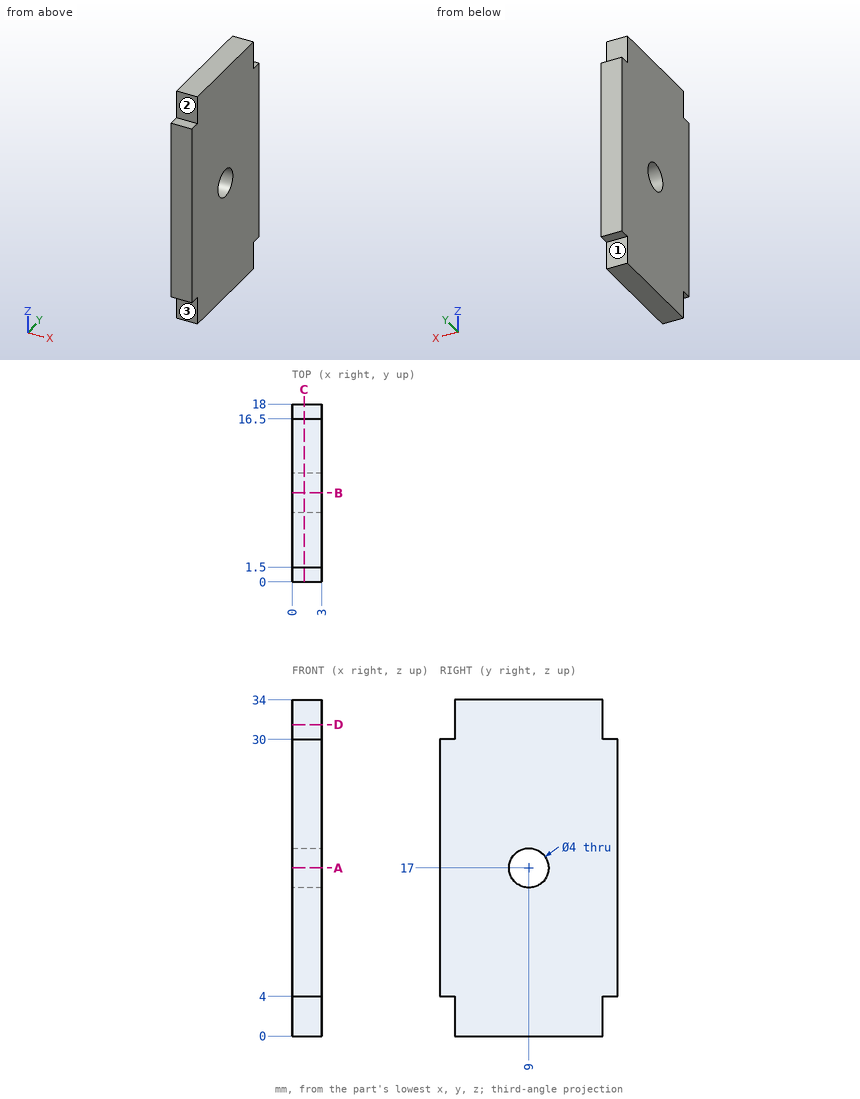
Drawing for the job (mm, zero at the part's lowest x, y, z). A direction names the side the tool comes from. Round coordinates to 2 decimals unless told otherwise and drop trailing zeros. Write each loop counter-clockwise with the first axis right and the second up, starting at its lowest first coordinate (ties: lowest second). Pieces come first, ordered by that corner, then holes. Notation, with made-up numbers: M 52,14 L 75,14 A26 cw 75,38 Z; hole C -38,63 d2. An arc over 180 degrees is marked long. Answer as a JSON object with one key per item and string values. Group by question number.
(1) Drill centre lines: L1, parallel to Y at x = 0.9, z = 17; L2, parallel to Z at x = 2.8, y = 17.5; L3, parallel to Z at x = 0.85, y = 9.75. Where is each one in solid material? Low to high.
(2) Which spindle directions (+Z, -Z, +X, -X, +Y, -Y) get a long thin tool onto all of the face, cutting with end or side? Do the marked faces 1, 2 and 3. Say none if no direction does.
(3) Flat gauge pins, fed straight in: pin 1 (1.6 mm diameter, centred on x = 1, y = 17.5, fed in from +Z); pin 2 (1.2 mm diameter, centred on x = 2, y = 17.5, fed in from -Z); pin 3 (0.9 mm diameter, centred on x = 1, z = 31, fed in from +Y). Where does each tip first touch, or does it go through?
(4) Cut at B-B (y = 9). Give the cut face in (x, z), and give its area (3 significant figures).
(5) Cut at A-A (z = 17). Give the cut face in (x, y).
(6) Cut at D-D (z = 31.5). Give the cut face in (x, y).
(7) Cut at C-C (x = 1.2). Give the cut face in (y, z), and give its area (3 significant figures).
Responses:
{
 "1": {"L1": "y = 0 to 7, 11 to 18", "L2": "z = 4 to 30", "L3": "z = 0 to 15.15, 18.85 to 34"},
 "2": {"face 1": "-Z, +X, -X, +Y", "face 2": "+Z, +X, -X, -Y", "face 3": "-Z, +X, -X, -Y"},
 "3": {"pin 1": "stops at z = 30", "pin 2": "stops at z = 4", "pin 3": "stops at y = 16.5"},
 "4": {"outline": "M 0,0 L 3,0 L 3,15 L 0,15 Z; M 0,19 L 3,19 L 3,34 L 0,34 Z", "area": "90.0 mm2"},
 "5": {"outline": "M 0,0 L 3,0 L 3,7 L 0,7 Z; M 0,11 L 3,11 L 3,18 L 0,18 Z"},
 "6": {"outline": "M 0,1.5 L 3,1.5 L 3,16.5 L 0,16.5 Z"},
 "7": {"outline": "M 0,4 L 1.5,4 L 1.5,0 L 16.5,0 L 16.5,4 L 18,4 L 18,30 L 16.5,30 L 16.5,34 L 1.5,34 L 1.5,30 L 0,30 Z; hole C 9,17 d4", "area": "575 mm2"}
}
